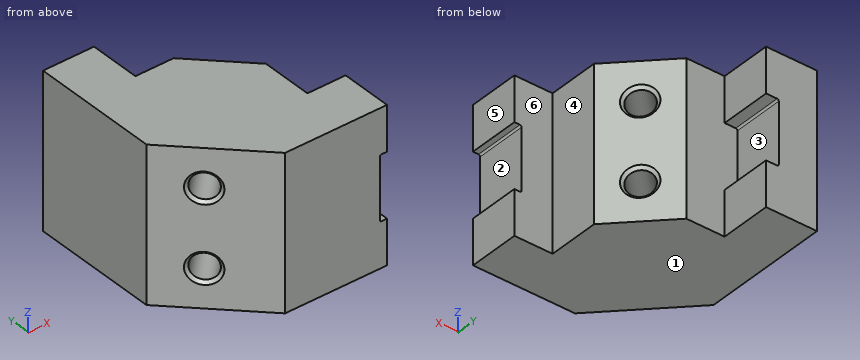
from build123d import *

# Parameters (mm, degrees)
BOSS_EXTRUDE1_DEPTH = 38.1
SKETCH2_R           = 6.35
CUT_EXTRUDE1_DEPTH  = 142.777171117
CHAMFER1_SIZE       = 1.524
SKETCH3_W           = 6.35
SKETCH3_H           = 31.75
CUT_EXTRUDE2_DEPTH  = 25.4
SKETCH4_W           = 3.590345221
SKETCH4_H           = 31.75
CUT_EXTRUDE3_DEPTH  = 124.131068378
FILLET1_R           = 0.8382


with BuildPart() as part:
    # Sketch1 → Boss-Extrude1 (new, symmetric)
    with BuildSketch(Plane.XY):
        Polygon((0, 0), (0, -63.5), (38.1, -101.6), (88.9, -101.6), (88.9, -76.2), (69.85, -76.2), (69.85, -50.8), (44.45, -25.4), (25.4, -25.4), (25.4, 0), align=None)
    extrude(amount=BOSS_EXTRUDE1_DEPTH, both=True)

    # Sketch2 → Cut-Extrude1 (cut, through all)
    with BuildSketch(Plane(origin=(9.525, 9.525, 0), x_dir=(0, 0, -1), z_dir=(0.7071067811865488, 0.7071067811865464, 0))):
        with Locations(Location((-19.05, -67.35463315, 0), (0, 0, 90))):
            Circle(SKETCH2_R)
        with Locations(Location((19.05, -67.35463315, 0), (0, 0, 90))):
            Circle(SKETCH2_R)
    extrude(amount=-CUT_EXTRUDE1_DEPTH, mode=Mode.SUBTRACT)

    # Chamfer1
    chamfer1_edges = [part.edges().sort_by_distance(p)[0] for p in [
        (20.367045905, -83.867045905, 19.05),
        (61.642045905, -42.592045905, 19.05),
        (20.367045905, -83.867045905, -19.05),
        (61.642045905, -42.592045905, -19.05),
    ]]
    chamfer(chamfer1_edges, length=CHAMFER1_SIZE)

    # Sketch3 → Cut-Extrude2 (cut)
    with BuildSketch(Plane(origin=(0, 0, 0), x_dir=(1, 0, 0), z_dir=(0, 1, 0))):
        with Locations((22.225, 0)):
            Rectangle(SKETCH3_W, SKETCH3_H)
    extrude(amount=-CUT_EXTRUDE2_DEPTH, mode=Mode.SUBTRACT)

    # Sketch4 → Cut-Extrude3 (cut, through all)
    with BuildSketch(Plane(origin=(0, -76.2, 0), x_dir=(1, 0, 0), z_dir=(0, 1, 0))):
        with Locations((87.10482739, 0)):
            Rectangle(SKETCH4_W, SKETCH4_H)
    extrude(amount=-CUT_EXTRUDE3_DEPTH, mode=Mode.SUBTRACT)

    # Fillet1
    fillet1_edges = [part.edges().sort_by_distance(p)[0] for p in [
        (19.05, -12.7, -15.875),
        (19.05, -12.7, 15.875),
        (85.309654779, -88.9, 15.875),
        (85.309654779, -88.9, -15.875),
    ]]
    fillet(fillet1_edges, radius=FILLET1_R)


solid = part.part
Verification items for the finished model (mm, model axes). Face numbers are marked on the shaded views. A direction names the side the tool comes from. Give positions to 0.01 mm unless a question says otherwise; leave off trailing zeros. Order: outer loops, then holes, each group sorted by start corner. A loop starts at its lowest first (then second) coordinate and runs counter-clockwise, first axis right, second up. Notation, with made-up numbers: M 6.25,69.5 L 41.25,69.5 A26 cw 41.25,105.5 Z; hole C -40,83 d11. An arc over 180 degrees is marked long. Answer as a JSON object with one key per item and string values. Group by question number.
1) Cross-section at C-C (x = 66.5). Enter the section's corners in (y, z), then the cut area to 3 significant figures.
2) Mould release check, pull along Z, two halves, no side actions. Record for the marked faces 1, 2, 3 and 4: released by +Z, released by -Z, zero draft, split by the parting line, or undercut.
3) Scan lines: line 1 along Z through (x, y) = (49.5, -48.5); line 2 along Z through (x, y) = (30.5, -73); line 3 along X through (y, z) = (-21, 35). Record each from-to range of solid material in increasing order. Write a range as [from, to].
4) Cross-section at A-A (y = -7.5). Enter the section's corners in (x, z) (3 decimals), then the cut area to 3 significant figures.
5) Access from +Z, -Z, +X, -X, +Y, -Y to the whole of each face (thin tool, end or side, straight path). Record for the marked faces 5 and 6.
6) Cross-section at D-D (x = 30). Give the number of separate pieces and of enclosed holes in the cut face, then the cut area to 3 significant figures.
7) Depth check by flat-ended pin: pin 1 Ø7.5 at (y, z) = (-95, -2.5) entering from +X; pin 2 Ø6.5 at (y, z) = (-17.5, -31) entering from +X; pin 3 Ø3 at (x, z) = (49.5, 25.5) entering from +Y. Enter the tip coordinate at first touch or a pass-through.
8) Cross-section at B-B (z = -0.5). Enter the section's corners in (x, y).
Result sheet:
{
 "1": {"outline": "M -101.6,-38.1 L -47.45,-38.1 L -47.45,38.1 L -101.6,38.1 Z", "area": "4,130 mm2"},
 "2": {"face 1": "released by -Z", "face 2": "undercut", "face 3": "undercut", "face 4": "zero draft"},
 "3": {"line 1": "z = [-38.1, -25.1], [-13, 13], [25.1, 38.1]", "line 2": "z = [-38.1, -21.56], [-16.54, 16.54], [21.56, 38.1]", "line 3": "x = [0, 25.4]"},
 "4": {"outline": "M 0,-38.1 L 25.4,-38.1 L 25.4,-15.875 L 19.888,-15.875 A0.838 cw 19.05,-15.037 L 19.05,15.037 A0.838 cw 19.888,15.875 L 25.4,15.875 L 25.4,38.1 L 0,38.1 Z", "area": "1,730 mm2"},
 "5": {"face 5": "+Z, -Z, +X, +Y, -Y", "face 6": "+Z, -Z, +X, +Y"},
 "6": {"separate pieces": "1", "enclosed holes": "2", "area": "4,830 mm2"},
 "7": {"pin 1": "stops at x = 85.31", "pin 2": "stops at x = 25.4", "pin 3": "stops at y = -28.95"},
 "8": {"outline": "M 0,-63.5 L 38.1,-101.6 L 85.31,-101.6 L 85.31,-76.2 L 69.85,-76.2 L 69.85,-50.8 L 44.45,-25.4 L 19.05,-25.4 L 19.05,0 L 0,0 Z"}
}
